Verification items for the finished model (mm, model axes). Face numbers are marked on the shaded views. A direction names the side the tool comes from. Round coordinates to 2 decimals unless told otherwise and drop trailing zeros. Order: outer loops, then holes, each group sorted by start corner. A loop starts at its lowest first (then second) coordinate and runs counter-clockwise, first axis right, second up. Notation, with made-up numbers: (38, 27) -> (54, 27) arc R20 cw to (54, 59) -> close; hole circle Ø1 at (-37, 28). An arc over 180 degrees is marked (long way). Put each result on its own line as item: value.
from build123d import *

# Parameters (mm, degrees)
SKETCH1_W           = 64
SKETCH1_H           = 30
BOSS_EXTRUDE1_DEPTH = 3
CUT_EXTRUDE1_REACH  = 72.746
SKETCH2_W           = 29
SKETCH2_H           = 12.5
SKETCH2_H_2         = 12
SKETCH2_W_2         = 20
SKETCH2_H_3         = 9.7
SKETCH2_W_3         = 30
SKETCH2_H_4         = 10.5
SKETCH3_W           = 64
SKETCH3_H           = 2.5
BOSS_EXTRUDE3_DEPTH = 5
CUT_EXTRUDE2_REACH  = 73.134
SKETCH4_R           = 1.419176597


with BuildPart() as part:
    # Sketch1 → Boss-Extrude1 (new body)
    with BuildSketch(Plane(origin=(0, 0, 0), x_dir=(1, 0, 0), z_dir=(0, 1, 0))):
        with Locations((32, 15)):
            Rectangle(SKETCH1_W, SKETCH1_H)
    extrude(amount=BOSS_EXTRUDE1_DEPTH)

    # Sketch2 → Cut-Extrude1 (cut, up to next)
    with BuildSketch(Plane(origin=(0, 3, 0), x_dir=(1, 0, 0), z_dir=(0, 1, 0)), mode=Mode.PRIVATE) as cut_extrude1_sk1:
        with Locations((16.5, 10.25)):
            Rectangle(SKETCH2_W, SKETCH2_H)
    cut_extrude1_tool1 = extrude(cut_extrude1_sk1.sketch, amount=-CUT_EXTRUDE1_REACH, mode=Mode.PRIVATE) & part.part
    # Sketch2 → Cut-Extrude1 (cut, up to next)
    with BuildSketch(Plane(origin=(0, 3, 0), x_dir=(1, 0, 0), z_dir=(0, 1, 0)), mode=Mode.PRIVATE) as cut_extrude1_sk2:
        with Locations((47.5, 21.7)):
            Rectangle(SKETCH2_W, SKETCH2_H_2)
    cut_extrude1_tool2 = extrude(cut_extrude1_sk2.sketch, amount=-CUT_EXTRUDE1_REACH, mode=Mode.PRIVATE) & part.part
    # Sketch2 → Cut-Extrude1 (cut, up to next)
    with BuildSketch(Plane(origin=(0, 3, 0), x_dir=(1, 0, 0), z_dir=(0, 1, 0)), mode=Mode.PRIVATE) as cut_extrude1_sk3:
        with Locations((52, 8.85)):
            Rectangle(SKETCH2_W_2, SKETCH2_H_3)
    cut_extrude1_tool3 = extrude(cut_extrude1_sk3.sketch, amount=-CUT_EXTRUDE1_REACH, mode=Mode.PRIVATE) & part.part
    # Sketch2 → Cut-Extrude1 (cut, up to next)
    with BuildSketch(Plane(origin=(0, 3, 0), x_dir=(1, 0, 0), z_dir=(0, 1, 0)), mode=Mode.PRIVATE) as cut_extrude1_sk4:
        with Locations((15, 24.75)):
            Rectangle(SKETCH2_W_3, SKETCH2_H_4)
    cut_extrude1_tool4 = extrude(cut_extrude1_sk4.sketch, amount=-CUT_EXTRUDE1_REACH, mode=Mode.PRIVATE) & part.part
    add(cut_extrude1_tool1.solids().sort_by_distance((16.5, 3, -10.25))[0], mode=Mode.SUBTRACT)
    add(cut_extrude1_tool2.solids().sort_by_distance((47.5, 3, -21.7))[0], mode=Mode.SUBTRACT)
    add(cut_extrude1_tool3.solids().sort_by_distance((52, 3, -8.85))[0], mode=Mode.SUBTRACT)
    add(cut_extrude1_tool4.solids().sort_by_distance((15, 3, -24.75))[0], mode=Mode.SUBTRACT)

    # Sketch3 → Boss-Extrude3 (add)
    with BuildSketch(Plane(origin=(0, 3, 0), x_dir=(1, 0, 0), z_dir=(0, 1, 0))):
        with Locations((32, 1.25)):
            Rectangle(SKETCH3_W, SKETCH3_H)
    extrude(amount=BOSS_EXTRUDE3_DEPTH)

    # Sketch4 → Cut-Extrude2 (cut, up to next)
    with BuildSketch(Plane.XY, mode=Mode.PRIVATE) as cut_extrude2_sk1:
        with Locations((61.5, 5.5)):
            Circle(SKETCH4_R)
    cut_extrude2_tool1 = extrude(cut_extrude2_sk1.sketch, amount=-CUT_EXTRUDE2_REACH, mode=Mode.PRIVATE) & part.part
    # Sketch4 → Cut-Extrude2 (cut, up to next)
    with BuildSketch(Plane.XY, mode=Mode.PRIVATE) as cut_extrude2_sk2:
        with Locations((4.5, 5.5)):
            Circle(SKETCH4_R)
    cut_extrude2_tool2 = extrude(cut_extrude2_sk2.sketch, amount=-CUT_EXTRUDE2_REACH, mode=Mode.PRIVATE) & part.part
    add(cut_extrude2_tool1.solids().sort_by_distance((61.5, 5.5, 0))[0], mode=Mode.SUBTRACT)
    add(cut_extrude2_tool2.solids().sort_by_distance((4.5, 5.5, 0))[0], mode=Mode.SUBTRACT)


solid = part.part
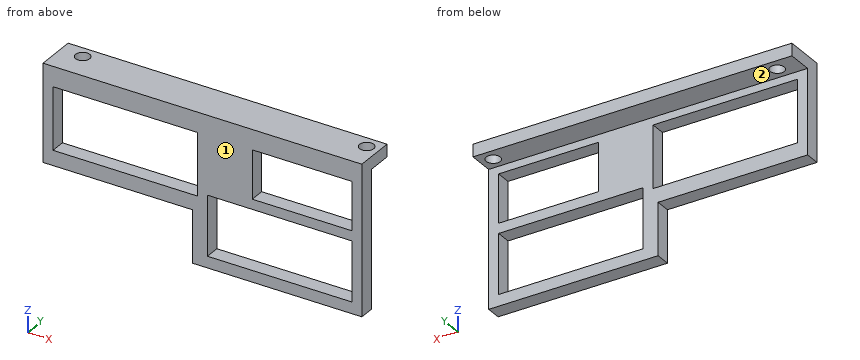
Item 1: Gauge pin test, flat ends, axial feed: pin 1 Ø3 at (x, y) = (23.5, 1.5) entering from -Z; pin 2 Ø3.5 at (y, z) = (1.5, -22) entering from -X; pin 3 Ø5 at (x, z) = (20.5, -8) entering from -Y; pin 4 Ø6 at (x, z) = (32.5, -26) entering from +Y. Record the tip position at first contact, or that the pin passes through.
Check sheet entries:
pin 1: stops at z = -19.5
pin 2: stops at x = 30
pin 3: passes through
pin 4: stops at y = 3
Item 2: Tool access check on the marked faces 1 and 2. Record the directions out of +Z, -Z, +X, -X, +Y, -Y that give a thin tool (end or side, any length) a straight path to the whole face; none if there is none.
Check sheet entries:
face 1: +Z, -Z, +X, -X, -Y
face 2: -Z, +X, -X, +Y
Item 3: Section check C-C on z = -24.75. Record the boundary of the cut face in (x, y), then the cut area to 3 significant figures.
Check sheet entries:
outline: (30, 0) -> (33, 0) -> (33, 3) -> (30, 3) -> close; (62, 0) -> (64, 0) -> (64, 3) -> (62, 3) -> close
area: 15.0 mm^2
Item 4: Section check B-B on z = -8.75. Record the boundary of the cut face in (x, y).
Check sheet entries:
outline: (0, 0) -> (2, 0) -> (2, 3) -> (0, 3) -> close; (31, 0) -> (42, 0) -> (42, 3) -> (31, 3) -> close; (62, 0) -> (64, 0) -> (64, 3) -> (62, 3) -> close
Item 5: Section check D-D on y = 4.75. Record the boundary of the cut face in (x, z), then the cut area to 3 significant figures.
Check sheet entries:
outline: (0, -2.5) -> (3.3, -2.5) -> (3.3, 0) -> (0, 0) -> close; (5.7, -2.5) -> (60.3, -2.5) -> (60.3, 0) -> (5.7, 0) -> close; (62.7, -2.5) -> (64, -2.5) -> (64, 0) -> (62.7, 0) -> close
area: 148 mm^2
Item 6: Section check A-A on x = 36. Record the boundary of the cut face in (y, z), then the cut area to 3 significant figures.
Check sheet entries:
outline: (0, -30) -> (3, -30) -> (3, -27.7) -> (0, -27.7) -> close; (0, -15.7) -> (3, -15.7) -> (3, -2.5) -> (8, -2.5) -> (8, 0) -> (0, 0) -> close
area: 66.5 mm^2
Item 7: Material ranges on L1, parallel to Y at x = 4.5, z = -0.55; L2, parallel to X at y = 1, z = -15.5; L3, parallel to Z at x = 33.5, y = 1.25, recorded low to high. Write a range as [from, to].
Check sheet entries:
L1: y = [0, 4.08], [6.92, 8]
L2: x = [0, 2], [31, 64]
L3: z = [-30, -27.7], [-15.7, 0]
